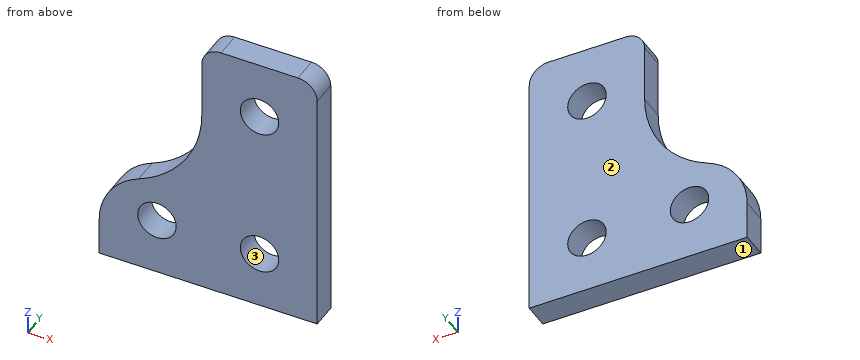
from build123d import *

# Parameters (mm, degrees)
F0_W      = 17
F0_H      = 15
F1_DEPTH  = 2
F2_R      = 1.5
F3_DEPTH  = 25
F4_W      = 9
F4_H      = 2
F5_DEPTH  = 6
F6_R      = 1.5
F7_DEPTH  = 25
F8_R      = 1.5
F9_W      = 17
F9_H      = 2
F10_DEPTH = 1
F11_W     = 17
F11_H     = 6
F12_DEPTH = 8
F13_W     = 17
F13_H     = 8
F14_DEPTH = 25
F15_W     = 17
F15_H     = 2
F16_DEPTH = 1
F17_R     = 8
F18_DEPTH = 25
F19_R     = 5


with BuildPart() as f1:
    # F0 (on Front) → F1 (new body)
    with BuildSketch(Plane.XZ):
        Rectangle(F0_W, F0_H)
    extrude(amount=F1_DEPTH)

    # F2 (on face) → F3 (cut)
    with BuildSketch(Plane.XZ.offset(2)):
        with Locations((-4, -3)):
            Circle(F2_R)
        with Locations((4, -3)):
            Circle(F2_R)
    extrude(amount=-F3_DEPTH, mode=Mode.SUBTRACT)

    # F4 (on face) → F5 (join)
    with BuildSketch(Plane.XY.offset(7.5)):
        with Locations((4, -1)):
            Rectangle(F4_W, F4_H)
    extrude(amount=F5_DEPTH)

    # F6 (on face) → F7 (cut)
    with BuildSketch(Plane.XZ.offset(2)):
        with Locations((4, 9)):
            Circle(F6_R)
    extrude(amount=-F7_DEPTH, mode=Mode.SUBTRACT)

    # F8
    f8_edges = [f1.edges().sort_by_distance(p)[0] for p in [
        (8.5, -1, 13.5),
        (-0.5, -1, 13.5),
    ]]
    fillet(f8_edges, radius=F8_R)

    # F9 (on face) → F10 (join)
    with BuildSketch(Plane(origin=(0, 0, -7.5), x_dir=(1, 0, 0), z_dir=(0, 0, -1))):
        with Locations((0, 1)):
            Rectangle(F9_W, F9_H)
    extrude(amount=F10_DEPTH)

    # F11 (on face) → F12 (join)
    with BuildSketch(Plane(origin=(0, 0, -8.5), x_dir=(1, 0, 0), z_dir=(0, 0, -1))):
        with Locations((0, -1)):
            Rectangle(F11_W, F11_H)
    extrude(amount=F12_DEPTH)

    # F13 (on face) → F14 (cut)
    with BuildSketch(Plane(origin=(0, 4, 0), x_dir=(-1, 0, 0), z_dir=(0, 1, 0))):
        with Locations((0, -12.5)):
            Rectangle(F13_W, F13_H)
    extrude(amount=-F14_DEPTH, mode=Mode.SUBTRACT)

    # F15 (on face) → F16 (cut)
    with BuildSketch(Plane(origin=(0, 0, -8.5), x_dir=(1, 0, 0), z_dir=(0, 0, -1))):
        with Locations((0, 1)):
            Rectangle(F15_W, F15_H)
    extrude(amount=-F16_DEPTH, mode=Mode.SUBTRACT)

    # F17 (on face) → F18 (cut)
    with BuildSketch(Plane(origin=(0, 0, 0), x_dir=(-1, 0, 0), z_dir=(0, 1, 0))):
        with Locations((8.5, 7.5)):
            Circle(F17_R)
    extrude(amount=-F18_DEPTH, mode=Mode.SUBTRACT)

    # F19
    f19_edges = [f1.edges().sort_by_distance(p)[0] for p in [
        (-8.5, -1, -0.5),
    ]]
    fillet(f19_edges, radius=F19_R)


solid = f1.part
Input: part model. Units: mm. Frame: model coordinates. Face numbers are marked on the shaded views. Coordinates: 2 decimals unless noted, no trailing zeros. Loops run counter-clockwise (first coordinate to the right, second up) from the corner with the lowest first, then second, coordinate; pieces in that order, holes last.
(1) Section C-C on y = -0.25. Return the cut outline in (x, z).
(2) Pull-direction query (Z, two-part tool) for the marked faces 1, 2 and 3; classes: released by +Z, released by -Z, zero draft, split by the parting line, or undercut.
(3) Material intervals for probe 1 along Z at (x, y) = (4, -1.2); probe 2 along X at (y, z) = (-0.45, -4); probe 3 along X at (y, z) = (-1.3, 10), sorted ascending.
(4) First-contact query: pin 1 Ø3.5 at (x, z) = (4, -3) entering from +Y. Flat tip, straight axial feed; report the tip coordinate or a pass-through.
(5) Section B-B on z = 9. Return the cut outline in (x, y).
(6) Section D-D on z = -4.25. Return the cut outline in (x, y).
(7) Section A-A on x = 4. Return the cut outline in (y, z), then the cut area to 3 significant figures.
Data:
1. outline: (-8.5, -7.5) - (8.5, -7.5) - (8.5, 12) arc R1.5 ccw to (7, 13.5) - (1, 13.5) arc R1.5 ccw to (-0.5, 12) - (-0.5, 7.5) arc R8 cw to (-5.42, 0.12) arc R5 ccw to (-8.5, -4.5) - close; hole circle Ø3 at (-4, -3); hole circle Ø3 at (4, -3); hole circle Ø3 at (4, 9)
2. face 1: released by -Z
2. face 2: zero draft
2. face 3: undercut
3. probe 1: z = -7.5 to -4.5, -1.5 to 7.5, 10.5 to 13.5
3. probe 2: x = -8.47 to -5.12, -2.88 to 2.88, 5.12 to 8.5
3. probe 3: x = -0.5 to 2.88, 5.12 to 8.5
4. pin 1: stops at y = 0
5. outline: (-0.5, -2) - (2.5, -2) - (2.5, 0) - (-0.5, 0) - close; (5.5, -2) - (8.5, -2) - (8.5, 0) - (5.5, 0) - close
6. outline: (-8.49, -2) - (-4.83, -2) - (-4.83, 0) - (-8.49, 0) - close; (-3.17, -2) - (3.17, -2) - (3.17, 0) - (-3.17, 0) - close; (4.83, -2) - (8.5, -2) - (8.5, 0) - (4.83, 0) - close
7. outline: (-2, -7.5) - (0, -7.5) - (0, -4.5) - (-2, -4.5) - close; (-2, -1.5) - (0, -1.5) - (0, 7.5) - (-2, 7.5) - close; (-2, 10.5) - (0, 10.5) - (0, 13.5) - (-2, 13.5) - close
7. area: 30.0 mm2
